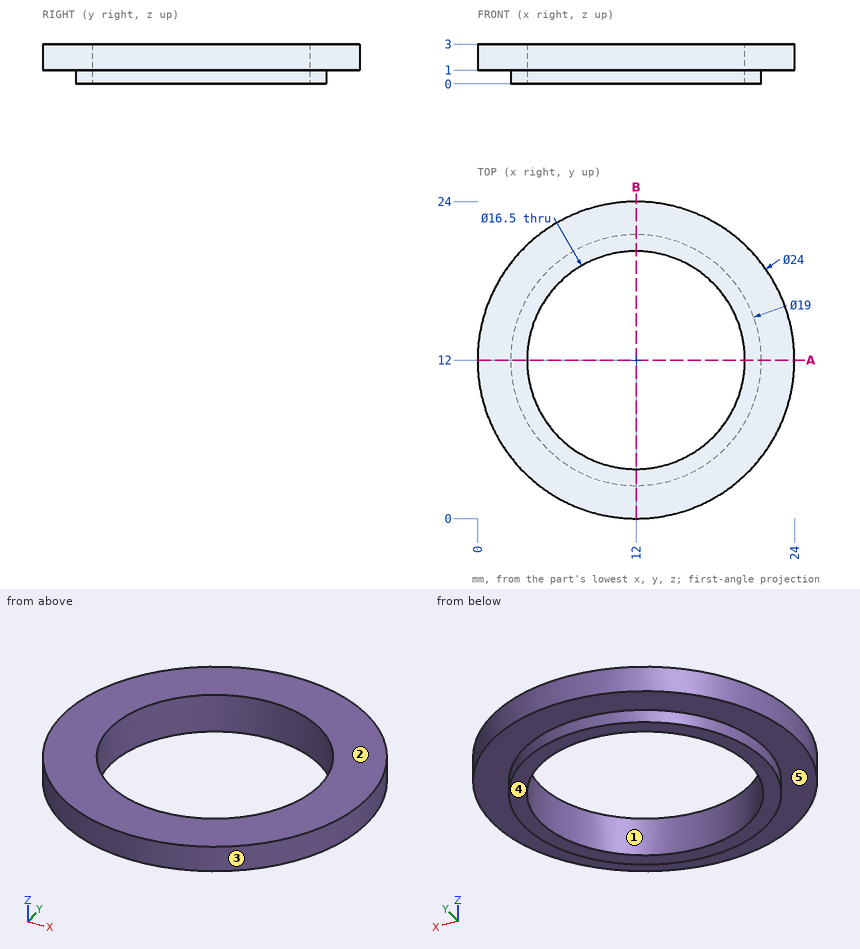
Answer from the drawing. Dimensions are ordinates in mm from the lowest x, y and z of the part. A direction names the side the tool comes from. Give positions to 0.01 mm unless a question says otherwise; leave off trailing zeros. Write each loop counter-clockwise with the first axis right and the second up, starting at its lowest first coordinate (ties: lowest second). Pieces come first, ordered by that corner, then holes. Notation, with made-up numbers: (21.25, 61) - (35.25, 61) arc R9 cw to (35.25, 65) - close; hole circle Ø11 at (87, 71). An arc over 180 degrees is marked (long way). Answer in a Markdown table with one row per item. Add a question column.
Item 1: Section A-A, the plane y = 12 is taken. Write down the section's boundary in (x, z).
Item 2: A tool of negligible diameter and unlimited length cuts with its end or side. For the marked faces 4 and 5, from which of +Z, -Z, +X, -X, +Y, -Y can it reach the whole face along a straight path? Write none if from no direction.
Item 3: Determine the mould class of the marked faces 1, 2 and 3 for opening direction X: pulls with the +X half, pulls with the -X half, needs draft (parallel to the pull), parting line crosses it, or undercut.
Item 4: A flat-ended cylindrical pin translates along its axis: P1, Ø1.5, axis at y = 18, z = 2, coming from the +X side. Find the tip coordinate at first contact, or state that the pin passes through.
Item 5: Find the intervals of material crossed by L1, parallel to Y at x = 12, z = 1.55; L2, parallel to Z at x = 5.5, y = 22; L3, parallel to Y at x = 12, z = 0.75, in increasing order.
Recorded:
| question | item | result |
|---|---|---|
| 1 | outline | (0, 1) - (2.5, 1) - (2.5, 0) - (3.75, 0) - (3.75, 3) - (0, 3) - close; (20.25, 0) - (21.5, 0) - (21.5, 1) - (24, 1) - (24, 3) - (20.25, 3) - close |
| 2 | face 4 | -Z, +X, -X, +Y, -Y |
| 2 | face 5 | -Z |
| 3 | face 1 | undercut |
| 3 | face 2 | needs draft |
| 3 | face 3 | parting line crosses it |
| 4 | P1 | stops at x = 22.79 |
| 5 | L1 | y = 0 to 3.75, 20.25 to 24 |
| 5 | L2 | z = 1 to 3 |
| 5 | L3 | y = 2.5 to 3.75, 20.25 to 21.5 |
